Geometry: final body of the model. Coordinates: model frame, mm. A direction names the side the tool comes from. Round coordinates to 2 decimals unless told otherwise and drop trailing zeros. Order: outer loops, then holes, each group sorted by start corner. A loop starts at its lowest first (then second) coordinate and runs counter-clockwise, first axis right, second up. Notation, with made-up numbers: (-2.5, 2.25) -> (45.5, 2.25) arc R22 ccw to (45.5, 34.25) -> close; hole circle Ø9 at (31, -13). An arc over 180 degrees is marked (long way). Put each result on its own line as item: value.
```python
from build123d import *

# Parameters (mm, degrees)
SALIENTE_EXTRUIR1_DEPTH = 4
SALIENTE_EXTRUIR2_START = 4.77
CROQUIS2_R              = 4
SALIENTE_EXTRUIR2_DEPTH = 4.77
CROQUIS3_R              = 2.2
SALIENTE_EXTRUIR3_DEPTH = 8.5
SALIENTE_EXTRUIR4_DEPTH = 2
CROQUIS5_R              = 2
SALIENTE_EXTRUIR5_DEPTH = 23
CROQUIS6_R              = 0.95
SALIENTE_EXTRUIR6_DEPTH = 2
CROQUIS7_R              = 2.65
CROQUIS7_R_2            = 0.95
SALIENTE_EXTRUIR7_DEPTH = 3
CROQUIS8_R              = 1.25
CORTAR_EXTRUIR1_DEPTH   = 0.5


with BuildPart() as part:
    # Croquis1 → Saliente-Extruir1 (new body)
    with BuildSketch(Plane.XY):
        with BuildLine():
            Line((0, 4), (50.4, 4))
            ThreePointArc((50.4, 4), (54.4, 0), (50.4, -4))
            Line((50.4, -4), (0, -4))
            ThreePointArc((0, -4), (-4, 0), (0, 4))
        make_face()
        with BuildLine():
            Line((-0.45, 2.459166525), (-0.45, 3.059166525))
            Line((-0.45, 3.059166525), (0.45, 3.059166525))
            Line((0.45, 3.059166525), (0.45, 2.459166525))
            ThreePointArc((0.45, 2.459166525), (0, -2.5), (-0.45, 2.459166525))
        make_face(mode=Mode.SUBTRACT)
    extrude(amount=-SALIENTE_EXTRUIR1_DEPTH)

    # Croquis2 → Saliente-Extruir2 (add)
    with BuildSketch(Plane.XY.offset(SALIENTE_EXTRUIR2_START)):
        Circle(CROQUIS2_R)
        with BuildLine():
            Line((-0.45, 3.059166525), (-0.45, 2.459166525))
            ThreePointArc((-0.45, 2.459166525), (0, -2.5), (0.45, 2.459166525))
            Line((0.45, 2.459166525), (0.45, 3.059166525))
            Line((0.45, 3.059166525), (-0.45, 3.059166525))
        make_face(mode=Mode.SUBTRACT)
    extrude(amount=-SALIENTE_EXTRUIR2_DEPTH)

    # Croquis3 → Saliente-Extruir3 (add)
    with BuildSketch(Plane.XY):
        with Locations((50.4, 0)):
            Circle(CROQUIS3_R)
    extrude(amount=SALIENTE_EXTRUIR3_DEPTH)

    # Croquis4 → Saliente-Extruir4 (add)
    with BuildSketch(Plane.XY.offset(8.5)):
        with BuildLine():
            Line((47.75, 15.5), (47.75, 0))
            ThreePointArc((47.75, 0), (50.4, -2.65), (53.05, 0))
            Line((53.05, 0), (53.05, 15.5))
            ThreePointArc((53.05, 15.5), (50.4, 18.15), (47.75, 15.5))
        make_face()
    extrude(amount=SALIENTE_EXTRUIR4_DEPTH)

    # Croquis5 → Saliente-Extruir5 (add)
    with BuildSketch(Plane.XY.offset(10.5)):
        with Locations((50.4, 15.5)):
            Circle(CROQUIS5_R)
    extrude(amount=SALIENTE_EXTRUIR5_DEPTH)

    # Croquis6 → Saliente-Extruir6 (add)
    with BuildSketch(Plane.XY.offset(33.5)):
        with BuildLine():
            Line((47.75, 15.5), (47.75, 0))
            ThreePointArc((47.75, 0), (50.4, -2.65), (53.05, 0))
            Line((53.05, 0), (53.05, 15.5))
            ThreePointArc((53.05, 15.5), (50.4, 18.15), (47.75, 15.5))
        make_face()
        with Locations((50.4, 0)):
            Circle(CROQUIS6_R, mode=Mode.SUBTRACT)
    extrude(amount=SALIENTE_EXTRUIR6_DEPTH)

    # Croquis7 → Saliente-Extruir7 (add)
    with BuildSketch(Plane.XY.offset(35.5)):
        with Locations((50.4, 0)):
            Circle(CROQUIS7_R)
        with Locations((50.4, 0)):
            Circle(CROQUIS7_R_2, mode=Mode.SUBTRACT)
    extrude(amount=SALIENTE_EXTRUIR7_DEPTH)

    # Croquis8 → Cortar-Extruir1 (cut)
    with BuildSketch(Plane(origin=(0, 0, 33.5), x_dir=(-1, 0, 0), z_dir=(0, 0, -1))):
        with Locations((-50.4, 0)):
            Circle(CROQUIS8_R)
    extrude(amount=-CORTAR_EXTRUIR1_DEPTH, mode=Mode.SUBTRACT)


solid = part.part
```
1. Cut plane B-B on y = 14.75. Return loops of the section in (x, z), and give its area (3 significant figures).
Ans:
outline: (47.75, 8.5) -> (53.05, 8.5) -> (53.05, 10.5) -> (52.25, 10.5) -> (52.25, 33.5) -> (53.05, 33.5) -> (53.05, 35.5) -> (47.75, 35.5) -> (47.75, 33.5) -> (48.55, 33.5) -> (48.55, 10.5) -> (47.75, 10.5) -> close
area: 106 mm²
2. Material intervals for probe 1 along X at (y, z) = (0, -2.2); probe 2 along Y at (x, z) = (50.4, 33.75); probe 3 along Y at (x, z) = (0, -1), sorted ascending.
Ans:
probe 1: -4 to -2.5, 2.5 to 54.4
probe 2: -2.65 to -1.25, 1.25 to 18.15
probe 3: -4 to -2.5, 3.06 to 4
3. Cut plane C-C on x = 19.5. Return loops of the section in (y, z), and give its area (3 significant figures).
Ans:
outline: (-4, -4) -> (4, -4) -> (4, 0) -> (-4, 0) -> close
area: 32.0 mm²
4. Contact query for flat-ended pins moving along their axis: P1, Ø1.6, axis at x = 49.5, y = 8, coming from the +Z side; P2, Ø12, axis at x = 15, y = -1, coming from the +Z side; P3, Ø0.5, axis at y = 2.5, z = 3, coming from the +X side. Output: stop coordinate, or through.
Ans:
P1: z = 35.5
P2: z = 0
P3: x = 3.31
5. Set-up query: faces 1 (the face through (54.4, 0.1, -2)), 2 (the face through (49.45, 0.04, 36.22)), 3 (the face through (50.34, -2.65, 9.49)), 4 (the face through (47.75, 8, 9)), 5 (the face through (53.05, 8, 9)). Return all of +Z, -Z, +X, -X, +Y, -Y with unobstructed straight access to the full face (end or side cutting, diameter ignored); none if empty.
Ans:
face 1: -Z, +X
face 2: +Z
face 3: +Z, -Y
face 4: +Z, -X, +Y, -Y
face 5: +Z, +X, +Y, -Y
6. Draft query along Z for faces 6 (the face through (50, 6, 10.5)), 7 (the face through (-2, -2, 4.77)), 8 (the face through (26, -4, -2)). Return one class per face: +Z half, -Z half, draft (parallel to the pull), parting line (faces both ways), or undercut.
Ans:
face 6: undercut
face 7: +Z half
face 8: draft
7. Cut plane A-A on y = 8. Return loops of the section in (x, z), and give its area (3 significant figures).
Ans:
outline: (47.75, 8.5) -> (53.05, 8.5) -> (53.05, 10.5) -> (47.75, 10.5) -> close; (47.75, 33.5) -> (53.05, 33.5) -> (53.05, 35.5) -> (47.75, 35.5) -> close
area: 21.2 mm²
